```python
from build123d import *

# Parameters (mm, degrees)
F1_DEPTH = 40


with BuildPart() as f1:
    # F0 (on Right) → F1 (new body)
    with BuildSketch(Plane.YZ):
        with BuildLine():
            add(Edge.make_bspline(
                [(-44.838704501, -6.3841724768), (-46.8453205455, -5.825457283), (-55.6681341229, -5.7726866527), (-57.7306464731, -1.4179735635), (-58.7613759126, 0)],
                knots=[0, 0, 0, 0, 0.5626960778, 1, 1, 1, 1], degree=3))
            Line((-44.838704501, -6.3841724768), (69.161295499, -6.3841724768))
            add(Edge.make_bspline(
                [(69.161295499, -6.3841724768), (71.4475678954, -6.1729190484), (74.6946425338, -5.8699737813), (81.8275271025, -0.1960649024), (84.2715006558, 8.1620243826), (80.7845015237, 18.3321377417), (81.6652249495, 21.4803665876)],
                knots=[0, 0, 0, 0, 0.0810771817, 0.1783295809, 0.2792067504, 0.4028908662, 0.4028908662, 0.4028908662, 0.4028908662], degree=3))
            add(Edge.make_bspline(
                [(81.6374216797, 22.4453190982), (81.6500654198, 22.1293211952), (81.6576451847, 21.8048438914), (81.6652249495, 21.4803665876)],
                knots=[0.9139943138, 0.9139943138, 0.9139943138, 0.9139943138, 1, 1, 1, 1], degree=3))
            add(Edge.make_bspline(
                [(75.7401209274, 23.3199857175), (78.0850621891, 23.5805863979), (81.1237295684, 23.990384777), (81.6374216797, 22.4453190982)],
                knots=[0.7859721691, 0.7859721691, 0.7859721691, 0.7859721691, 0.9689675221, 0.9689675221, 0.9689675221, 0.9689675221], degree=3))
            add(Edge.make_bspline(
                [(47.8096007504, 26.4636462757), (50.4151132719, 25.2566612425), (54.0270677376, 23.6070629686), (68.3082992802, 22.7847875979), (72.6222400219, 22.9734858293), (75.7401209274, 23.3199857175)],
                knots=[0, 0, 0, 0, 0.2310309702, 0.5426578797, 0.7859721691, 0.7859721691, 0.7859721691, 0.7859721691], degree=3))
            add(Edge.make_bspline(
                [(47.8096007504, 26.4636462757), (38.9469496949, 27.2014516696), (19.8383470871, 30.9230949853), (7.2381034379, 33.4919049177)],
                knots=[0.7500808852, 0.7500808852, 0.7500808852, 0.7500808852, 0.9114828872, 0.9114828872, 0.9114828872, 0.9114828872], degree=3))
            add(Edge.make_bspline(
                [(7.2381034379, 33.4919049177), (7.0293313069, 33.4424692791), (-0.6619575082, 31.5703885813), (-15.3393975904, 24.8264789662), (-19.5332629376, 21.2280452336), (-24.5166032072, 20.1923100725)],
                knots=[0.4361701211, 0.4361701211, 0.4361701211, 0.4361701211, 0.4414328852, 0.6293645181, 0.7611494878, 0.7611494878, 0.7611494878, 0.7611494878], degree=3))
            add(Edge.make_bspline(
                [(-24.5166032072, 20.1923100725), (-27.1952683602, 19.5284516677), (-30.5343573496, 19.1890804899), (-33.9337619399, 18.8384775563)],
                knots=[0, 0, 0, 0, 0.1548207433, 0.1548207433, 0.1548207433, 0.1548207433], degree=3))
            add(Edge.make_bspline(
                [(-33.9337619399, 18.8384775563), (-36.1619029939, 18.5738236368), (-38.5117720873, 18.2998204972), (-40.8694513595, 17.9847684884)],
                knots=[0.82699703, 0.82699703, 0.82699703, 0.82699703, 0.867474623, 0.867474623, 0.867474623, 0.867474623], degree=3))
            add(Edge.make_bspline(
                [(-40.8694513595, 17.9847684884), (-41.7301591235, 17.843002501), (-47.4822650158, 16.7449192121), (-54.3846967183, 12.8459477913), (-60.8683867647, 6.2520742648), (-59.4702371494, 1.5500023351), (-58.7613759126, 0)],
                knots=[0.2618071145, 0.2618071145, 0.2618071145, 0.2618071145, 0.3034989867, 0.5490089029, 0.7603362688, 0.8611758874, 0.8611758874, 0.8611758874, 0.8611758874], degree=3))
        make_face()
        with BuildLine():
            add(Edge.make_bspline(
                [(10.9806247056, 29.136126861), (7.2108730674, 28.4910239279), (-0.4322852797, 26.9914683958), (-17.0990938919, 21.1353577397), (-11.5334123789, 17.4561242614), (-11.4637765201, 17.4852853631), (-11.4568779245, 17.4886267632)],
                knots=[0, 0, 0, 0, 0.3909237382, 0.7850289694, 0.9782824352, 1, 1, 1, 1], degree=3))
            add(Edge.make_bspline(
                [(35.6915146112, 17.4886267632), (36.7587346212, 17.9547515009), (47.3920951695, 20.4782306051), (31.2295468414, 28.9607742297), (18.3165498499, 29.9648338159), (10.9806247056, 29.136126861)],
                knots=[0, 0, 0, 0, 0.2520150835, 0.5614741686, 1, 1, 1, 1], degree=3))
            Line((35.6915146112, 17.4886267632), (21.6614138335, 17.4886267632))
            Line((21.6614138335, 17.4886267632), (-11.4568779245, 17.4886267632))
        make_face(mode=Mode.SUBTRACT)
        with BuildLine():
            add(Edge.make_bspline(
                [(-33.9337619399, 18.8384775563), (-36.2828655116, 18.5961990685), (-38.6607714567, 18.3485571057), (-40.8694513595, 17.9847684884)],
                knots=[0.1548207433, 0.1548207433, 0.1548207433, 0.1548207433, 0.2618071145, 0.2618071145, 0.2618071145, 0.2618071145], degree=3))
            add(Edge.make_bspline(
                [(-33.9337619399, 18.8384775563), (-36.1619029939, 18.5738236368), (-38.5117720873, 18.2998204972), (-40.8694513595, 17.9847684884)],
                knots=[0.82699703, 0.82699703, 0.82699703, 0.82699703, 0.867474623, 0.867474623, 0.867474623, 0.867474623], degree=3))
        make_face()
        with BuildLine():
            add(Edge.make_bspline(
                [(47.8096007504, 26.4636462757), (38.9469496949, 27.2014516696), (19.8383470871, 30.9230949853), (7.2381034379, 33.4919049177)],
                knots=[0.7500808852, 0.7500808852, 0.7500808852, 0.7500808852, 0.9114828872, 0.9114828872, 0.9114828872, 0.9114828872], degree=3))
            add(Edge.make_bspline(
                [(47.8096007504, 26.4636462757), (45.3407789538, 28.0318315658), (40.389939725, 31.0970656548), (25.1323891576, 35.0557908721), (13.8550573864, 35.0587488343), (7.2381034379, 33.4919049177)],
                knots=[0, 0, 0, 0, 0.1156638206, 0.269368798, 0.4361701211, 0.4361701211, 0.4361701211, 0.4361701211], degree=3))
        make_face()
        with BuildLine():
            add(Edge.make_bspline(
                [(75.7401209274, 23.3199857175), (78.0850621891, 23.5805863979), (81.1237295684, 23.990384777), (81.6374216797, 22.4453190982)],
                knots=[0.7859721691, 0.7859721691, 0.7859721691, 0.7859721691, 0.9689675221, 0.9689675221, 0.9689675221, 0.9689675221], degree=3))
            add(Edge.make_bspline(
                [(75.7401209274, 23.3199857175), (77.7663103657, 24.605784142), (81.2120858063, 26.792436855), (81.582065434, 23.8288066823), (81.6374216797, 22.4453190982)],
                knots=[0, 0, 0, 0, 0.5374481469, 0.9139943138, 0.9139943138, 0.9139943138, 0.9139943138], degree=3))
        make_face()
    extrude(amount=F1_DEPTH)


solid = f1.part
```
Check sheet for the modelled part. Datum: model origin and axes. Units: mm. Coordinates: 2 decimals unless noted, no trailing zeros. Write item = value, one per line. Start each with the question number.
1) Go/stop test with flat-tipped pins: P1, Ø3, axis at x = 25.5, y = 44.5, coming from the +Z side; P2, Ø1, axis at x = 18.5, z = 3, coming from the +Y side; P3, Ø8, axis at x = 26.5, y = -45.5, coming from the +Z side. Record where each tip stops, or that it passes through.
2) Mould release check, pull along Z, two halves, no side actions. Record for faces 1 (the flat face through (20, 11, -6.384)), 2 (the flat face through (20, 12, 17.489)), 3 (the flat face through (0, 13, 10)): +Z half, -Z half, draft (parallel to the pull), parting line (faces both ways), or undercut.
3) Material ranges on L1, parallel to Z at x = 12, y = 16; L2, parallel to Z at x = 10.5, y = 35; L3, parallel to Z at x = 9, y = 50, recorded low to high.
Ans:
q1.P1 = 29.3
q1.P2 = 82.62
q1.P3 = 17.88
q2.face_1 = -Z half
q2.face_2 = undercut
q2.face_3 = draft
q3.L1 = -6.38 to 17.49, 29.48 to 34.74
q3.L2 = -6.38 to 17.49, 26.3 to 32.33
q3.L3 = -6.38 to 25.47
